from build123d import *

# Parameters (mm, degrees)
SKETCH_1_R               = 10.2
SKETCH_1_R_2             = 4.2
SKETCH_1_R_3             = 1.5
EXTRUDE_1_DEPTH          = 1.5
SKETCH_2_R               = 5.8
SKETCH_2_R_2             = 4.2
EXTRUDE_2_DEPTH          = 15
FILLET_1_R               = 2
CUT_EXTRUDE_1_DEPTH      = 22.916432191
CUT_EXTRUDE_1_DEPTH_BACK = 22.916432191
SKETCH_3_R               = 1.5


with BuildPart() as part:
    # Эскиз1 → Бобышка-Вытянуть1 (new, symmetric)
    with BuildSketch(Plane.XY):
        Circle(SKETCH_1_R)
        Circle(SKETCH_1_R_2, mode=Mode.SUBTRACT)
        with Locations((0, 7.75)):
            Circle(SKETCH_1_R_3, mode=Mode.SUBTRACT)
        with Locations((-5.480077554, -5.480077554)):
            Circle(SKETCH_1_R_3, mode=Mode.SUBTRACT)
        with Locations(Location((5.480077554, -5.480077554, 0), (0, 0, 180))):
            Circle(SKETCH_1_R_3, mode=Mode.SUBTRACT)
    extrude(amount=EXTRUDE_1_DEPTH, both=True)

    # Эскиз2 → Бобышка-Вытянуть2 (add)
    with BuildSketch(Plane.XY.offset(1.5)):
        Circle(SKETCH_2_R)
        Circle(SKETCH_2_R_2, mode=Mode.SUBTRACT)
    extrude(amount=EXTRUDE_2_DEPTH)

    # Скругление1
    # the kernel refuses this fillet: 2 mm, written as the material it adds along each edge
    with BuildSketch(Plane(origin=(0, 0, 1.5), x_dir=(1, 0, 0), z_dir=(0, -1, 0))) as fillet_1_piece_1_section:
        with BuildLine():
            CenterArc((5.8 + FILLET_1_R, FILLET_1_R), FILLET_1_R, 180, 90)
            Line((5.8, FILLET_1_R), (5.8, 0))
            Line((5.8, 0), (5.8 + FILLET_1_R, 0))
        make_face()
    fillet_1_piece_1 = revolve(axis=Axis((0, 0, 1.5), (0, 0, 1)), mode=Mode.PRIVATE)
    fillet_1_piece_1 = fillet_1_piece_1 - Plane(origin=(-5.480077554, -5.480077554, 2.062024649), x_dir=(1, 0, 0), z_dir=(0, 0, -1)) * Cylinder(1.5, 32, mode=Mode.PRIVATE)
    fillet_1_piece_1 = fillet_1_piece_1 - Plane(origin=(5.480077554, -5.480077554, 2.062024649), x_dir=(-1, 0, 0), z_dir=(0, 0, -1)) * Cylinder(1.5, 32, mode=Mode.PRIVATE)
    fillet_1_piece_1 = fillet_1_piece_1 - Plane(origin=(0, 7.75, 2.062024649), x_dir=(1, 0, 0), z_dir=(0, 0, -1)) * Cylinder(1.5, 32, mode=Mode.PRIVATE)
    add(fillet_1_piece_1)

    # Эскиз3 → Вырез-Вытянуть1 (cut, two sides: drawn at the far end of the back side and taken through both)
    with BuildSketch(Plane(origin=(0, 0, 0), x_dir=(1, 0, 0), z_dir=(0, 1, 0)).offset(-CUT_EXTRUDE_1_DEPTH_BACK)):
        with Locations(Location((0, -10, 0), (0, 0, 270))):
            Circle(SKETCH_3_R)
    extrude(amount=CUT_EXTRUDE_1_DEPTH + CUT_EXTRUDE_1_DEPTH_BACK, mode=Mode.SUBTRACT)


solid = part.part
The listing builds one solid part. Answer for the finished solid, in the listing's coordinates (mm). A direction names the side the tool comes from. Coordinates: 2 decimals unless noted, no trailing zeros. Write each loop counter-clockwise with the first axis right and the second up, starting at its lowest first coordinate (ties: lowest second). Pieces come first, ordered by that corner, then holes. Notation, with made-up numbers: (28.5, -35) -> (70.5, -35) arc R11 ccw to (70.5, -22) -> close; hole circle Ø7 at (22.5, 34.25). An arc over 180 degrees is marked (long way). One line per question, with ' | ' between items.
1. Section C-C (z = 10) is taken. Determine the outline of the cut face in (x, y), and give its area (3 significant figures).
Verdict:
outline: (-1.5, -5.6) -> (-1.5, -3.92) arc R4.2 cw to (-1.5, 3.92) -> (-1.5, 5.6) arc R5.8 ccw to start; (1.5, -5.6) arc R5.8 ccw to (1.5, 5.6) -> (1.5, 3.92) arc R4.2 cw to (1.5, -3.92) -> close | area: 40.5 mm^2
2. Given pin 1 Ø5 at (x, y) = (0, 0) entering from +Z; pin 2 Ø1 at (x, z) = (-3.5, 8.5) entering from +Y; pin 3 Ø4 at (x, z) = (-6, 11.5) entering from -Y; pin 4 Ø5 at (y, z) = (2.5, 7) entering from -X, each flat-ended and moving along its own axis, determine where each tip first touches the part or whether it passes through.
Verdict:
pin 1: passes through | pin 2: stops at y = 4.96 | pin 3: stops at y = -4.2 | pin 4: stops at x = -5.8
3. Section D-D (z = 13.25) is taken. Determine the outline of the cut face in (x, y).
Verdict:
outline: circle Ø11.6 at (0, 0); hole circle Ø8.4 at (0, 0)
4. For a pull along X with two mould halves and no side action, classify faces 3 (the flat face through (4.4, 0.1, -1.5)), 4 (the cylindrical face through (-0.195, 6.263, -0.073)), 5 (the cylindrical face through (5.532, 1.742, 9.909)) as released by +X, released by -X, zero draft, split by the parting line, or undercut.
Verdict:
face 3: zero draft | face 4: undercut | face 5: split by the parting line
5. Section A-A (x = 0) is taken. Determine the outline of the cut face in (y, z), and give its area (3 significant figures).
Verdict:
outline: (-10.2, -1.5) -> (-4.2, -1.5) -> (-4.2, 8.5) -> (-5.8, 8.5) -> (-5.8, 3.5) arc R2 cw to (-7.8, 1.5) -> (-10.2, 1.5) -> close; (-5.8, 11.5) -> (-4.2, 11.5) -> (-4.2, 16.5) -> (-5.8, 16.5) -> close; (4.2, -1.5) -> (6.25, -1.5) -> (6.25, 2.24) arc R2 cw to (5.8, 3.5) -> (5.8, 8.5) -> (4.2, 8.5) -> close; (4.2, 11.5) -> (5.8, 11.5) -> (5.8, 16.5) -> (4.2, 16.5) -> close; (9.25, -1.5) -> (10.2, -1.5) -> (10.2, 1.5) -> (9.25, 1.5) -> close | area: 66.8 mm^2
6. Straight lines are drawn through the part: line 1 (Y direction, x = 0, z = 0.1); line 2 (Y direction, x = 0, z = 11.75); line 3 (Z direction, x = -5.5, y = 6.25). For each, find the intervals that lie inside material, in ascending order.
Verdict:
line 1: y = -10.2 to -4.2, 4.2 to 6.25, 9.25 to 10.2 | line 2: y = -5.8 to -4.2, 4.2 to 5.8 | line 3: z = -1.5 to 1.5
7. Which of the six approach directions +Z, -Z, +X, -X, +Y, -Y give full straight-line access (tool end or side, diameter ignored) to faces 1 (the flat face through (4, 2, 16.5)), 2 (the flat face through (2, -8, 1.5))?
Verdict:
face 1: +Z, +X, -X, +Y, -Y | face 2: +Z
8. Section B-B (y = 0) is taken. Determine the outline of the cut face in (x, z), and give its area (3 significant figures).
Verdict:
outline: (-10.2, -1.5) -> (-4.2, -1.5) -> (-4.2, 16.5) -> (-5.8, 16.5) -> (-5.8, 3.5) arc R2 cw to (-7.8, 1.5) -> (-10.2, 1.5) -> close; (4.2, -1.5) -> (10.2, -1.5) -> (10.2, 1.5) -> (7.8, 1.5) arc R2 cw to (5.8, 3.5) -> (5.8, 16.5) -> (4.2, 16.5) -> close | area: 85.7 mm^2
